Source: CAD feature listing. Evaluate the final solid. Frame: model axes, mm. A direction names the side the tool comes from. Round coordinates to 2 decimals unless told otherwise and drop trailing zeros. Loops run counter-clockwise (first coordinate to the right, second up) from the corner with the lowest first, then second, coordinate; pieces in that order, holes last.
(1) Set-up query: faces 1 (the flat face through (1.27, 13, 0)), 2 (the cylindrical face through (-4.49, 0.63, 0.24)). Return all of +Z, -Z, +X, -X, +Y, -Y with unobstructed straight access to the full face (end or side cutting, diameter ignored); none if empty.
(2) Mould query, pull axis Z, two halves, no side actions, for faces 3 (the flat face through (0, 0, 0)), 4 (the flat face through (10.904, 13.166, 2.504)), 5 (the flat face through (0, 13, -6.35)). Classes: pulls with the +Z half, pulls with the -Z half, needs draft (parallel to the pull), parting line crosses it, or undercut.
(3) First-contact query: pin 1 Ø1 at (y, z) = (20.5, -2) entering from -X; pin 2 Ø1.5 at (x, z) = (-5.08, 0) entering from +Y; pin 3 Ø1.1 at (x, z) = (6.35, -2.54) entering from +Y; pin 4 Ø6 at (y, z) = (7, -5) entering from -X. Flat tips, straight axial feed; report the tip coordinate or a pass-through.
(4) Section B-B, the plane y = 9.75. Return the cut outline in (x, z).
(5) Material intervals for probe 1 along X at (y, z) = (0.65, 0) (3 decimals); probe 2 along X at (y, z) = (14.5, 0); probe 3 along Z at (x, y) = (2.25, 17.5), sorted ascending.
(6) Section D-D, the plane z = -2.54. Return the cut outline in (x, y) (3 decimals).
(7) Section C-C, the plane x = -6.35. Return the cut outline in (y, z).
(8) Section A-A, the plane x = 6.35. Return the cut outline in (y, z) (3 decimals).
```python
from build123d import *

# Parameters (mm, degrees)
SKETCH1_R           = 5.08
BOSS_EXTRUDE4_DEPTH = 25.4
SKETCH1_9_R         = 5.08
SKETCH1_9_R_2       = 0.635
BOSS_EXTRUDE5_DEPTH = 1.27


with BuildPart() as part:
    # Sketch1 → Boss-Extrude4 (new body)
    with BuildSketch(Plane(origin=(0, 0, 0), x_dir=(1, 0, 0), z_dir=(0, 1, 0))):
        with BuildLine():
            Line((10.998522628, 6.35), (-7.775388174, 6.35))
            Line((-7.775388174, 6.35), (-10.998522628, 6.35))
            ThreePointArc((-10.998522628, 6.35), (-12.7, 0), (-10.998522628, -6.35))
            Line((-10.998522628, -6.35), (10.998522628, -6.35))
            ThreePointArc((10.998522628, -6.35), (12.267257994, -3.287001873), (12.7, 0))
            ThreePointArc((12.7, 0), (12.267257994, 3.287001873), (10.998522628, 6.35))
        make_face()
        with Locations((-6.35, 0)):
            Circle(SKETCH1_R, mode=Mode.SUBTRACT)
        Polygon((1.27, -5.08), (1.27, 0), (1.27, 5.08), (10.363946118, 5.08), (11.43, 0), (10.363946118, -5.08), align=None, mode=Mode.SUBTRACT)
    extrude(amount=BOSS_EXTRUDE4_DEPTH)

    # Sketch1_9 → Boss-Extrude5 (add)
    with BuildSketch(Plane(origin=(0, 0, 0), x_dir=(1, 0, 0), z_dir=(0, 1, 0))):
        with Locations((-6.35, 0)):
            Circle(SKETCH1_9_R)
        with Locations((-5.08, 0)):
            Circle(SKETCH1_9_R_2, mode=Mode.SUBTRACT)
        with Locations((-7.62, 0)):
            Circle(SKETCH1_9_R_2, mode=Mode.SUBTRACT)
        Polygon((1.27, 5.08), (1.27, 0), (1.27, -5.08), (10.363946118, -5.08), (11.43, 0), (10.363946118, 5.08), align=None)
        with Locations((3.528103699, 2.54)):
            Circle(SKETCH1_9_R_2, mode=Mode.SUBTRACT)
        with Locations((6.35, 2.54)):
            Circle(SKETCH1_9_R_2, mode=Mode.SUBTRACT)
        with Locations((9.202180779, 2.54)):
            Circle(SKETCH1_9_R_2, mode=Mode.SUBTRACT)
    extrude(amount=BOSS_EXTRUDE5_DEPTH)


solid = part.part
```
Output values:
1. face 1: +Y
1. face 2: +Y, -Y
2. face 3: needs draft
2. face 4: undercut
2. face 5: pulls with the -Z half
3. pin 1: stops at x = -12.61
3. pin 2: stops at y = 1.27
3. pin 3: passes through
3. pin 4: stops at x = -12.54
4. outline: (-11, -6.35) - (11, -6.35) arc R12.7 ccw to (11, 6.35) - (-11, 6.35) arc R12.7 ccw to start; hole circle Ø10.16 at (-6.35, 0); hole (1.27, -5.08) - (10.36, -5.08) - (11.43, 0) - (10.36, 5.08) - (1.27, 5.08) - close
5. probe 1: x = -12.7 to -8.255, -6.985 to -5.715, -4.445 to 12.7
5. probe 2: x = -12.7 to -11.43, -1.27 to 1.27, 11.43 to 12.7
5. probe 3: z = -6.35 to -5.08, 5.08 to 6.35
6. outline: (-12.443, 0) - (2.893, 0) - (2.893, 1.27) - (1.27, 1.27) - (1.27, 25.4) - (-1.951, 25.4) - (-1.951, 1.27) - (-10.749, 1.27) - (-10.749, 25.4) - (-12.443, 25.4) - close; (4.163, 0) - (5.715, 0) - (5.715, 1.27) - (4.163, 1.27) - close; (6.985, 0) - (8.567, 0) - (8.567, 1.27) - (6.985, 1.27) - close; (9.837, 0) - (12.443, 0) - (12.443, 25.4) - (10.897, 25.4) - (10.897, 1.27) - (9.837, 1.27) - close
7. outline: (0, -6.35) - (25.4, -6.35) - (25.4, -5.08) - (1.27, -5.08) - (1.27, 5.08) - (25.4, 5.08) - (25.4, 6.35) - (0, 6.35) - close
8. outline: (0, -6.35) - (25.4, -6.35) - (25.4, -5.08) - (1.27, -5.08) - (1.27, -3.175) - (0, -3.175) - close; (0, -1.905) - (1.27, -1.905) - (1.27, 5.08) - (25.4, 5.08) - (25.4, 6.35) - (0, 6.35) - close
